```python
from build123d import *

# Parameters (mm, degrees)
IZIM1_R                     = 1.5
Y_KSEKLIK_EKSTR_ZYON1_DEPTH = 72
RADYUS1_R                   = 0.5
RADYUS2_R                   = 0.5


with BuildPart() as part:
    # Çizim1 → Yükseklik-Ekstrüzyon1 (new body)
    with BuildSketch(Plane(origin=(0, 0, 0), x_dir=(1, 0, 0), z_dir=(0, 1, 0))):
        with Locations(Location((0, 0, 0), (0, 0, 270))):
            Circle(IZIM1_R)
    extrude(amount=Y_KSEKLIK_EKSTR_ZYON1_DEPTH)

    # Radyus1
    radyus1_edges = [part.edges().sort_by_distance(p)[0] for p in [
        (0, 72, -1.5),
    ]]
    fillet(radyus1_edges, radius=RADYUS1_R)

    # Radyus2
    radyus2_edges = [part.edges().sort_by_distance(p)[0] for p in [
        (0, 0, -1.5),
    ]]
    fillet(radyus2_edges, radius=RADYUS2_R)


solid = part.part
```
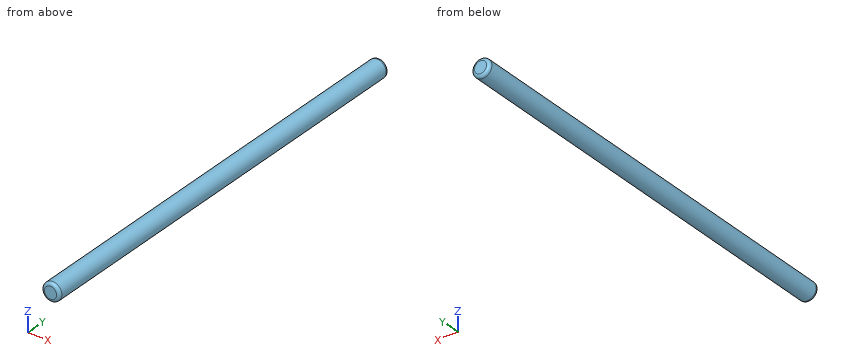
Model file for the job. Use its own axes, mm. Give positions to 0.01 mm unless a question says otherwise; leave off trailing zeros. Loops run counter-clockwise (first coordinate to the right, second up) from the corner with the lowest first, then second, coordinate; pieces in that order, holes last. Notation, with made-up numbers: (21.5, 55.25) -> (64.5, 55.25) arc R13 ccw to (64.5, 74.25) -> close; hole circle Ø11 at (75.5, 32). An arc over 180 degrees is marked (long way). Write each question's results on one line, items separated by ' | '.
(1) Probe line 1 along Y through (x, z) = (-0.95, -0.5); line 2 along Z through (x, y) = (-0.2, 32.5); line 3 along X through (y, z) = (24.5, -0.7). List the from-to ranges inside material, lowest first.
Geometry results:
line 1: y = 0.01 to 71.99 | line 2: z = -1.49 to 1.49 | line 3: x = -1.33 to 1.33
(2) Flat gauge pins, fed straight in: pin 1 Ø1.5 at (y, z) = (18.5, 0.5) entering from +X; pin 2 Ø1.5 at (x, y) = (1, 25.5) entering from -Z. Where does each tip first touch, or does it go through?
Geometry results:
pin 1: stops at x = 1.5 | pin 2: stops at z = -1.48
(3) Cut at A-A on y = 21. List the corners of the cut face in (x, z), and give its area (3 significant figures).
Geometry results:
outline: circle Ø3 at (0, 0) | area: 7.07 mm²
